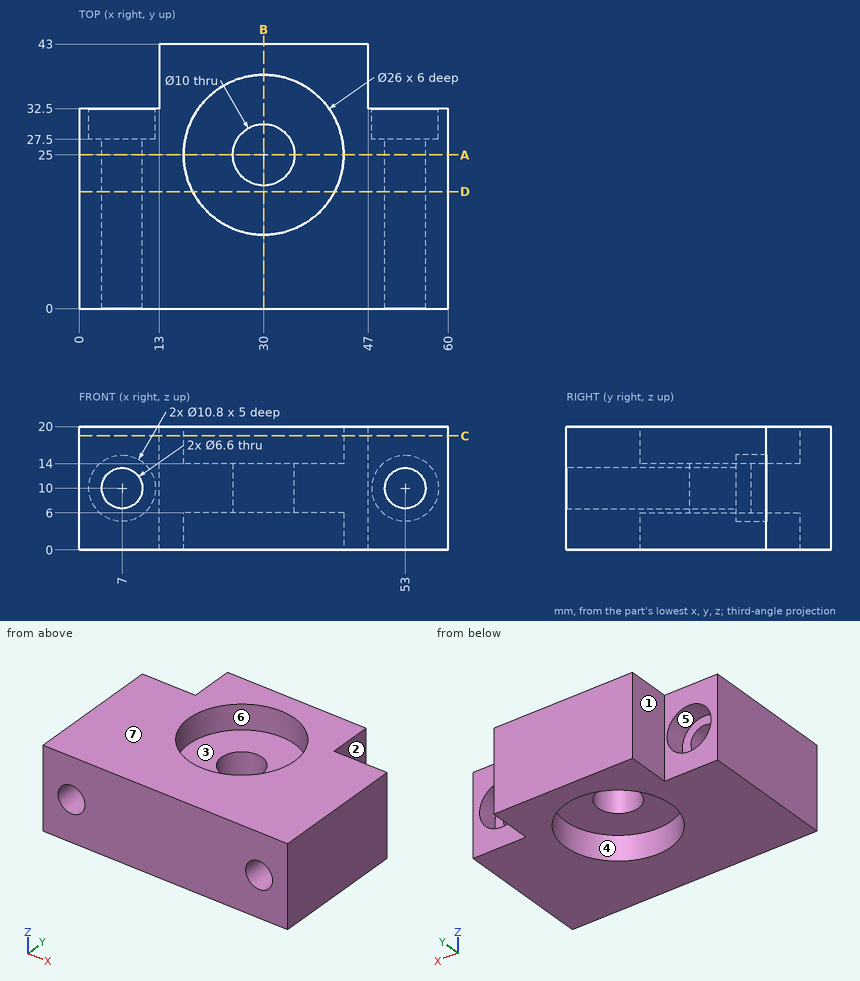
Design review of the part shown in the three views and the two pictorial views. Dimensions are in mm from the part's minimum x, y and z. A direction names the side the tool comes from. Round coordinates to 2 decimals unless told otherwise and drop trailing zeros. Order: outer loops, then holes, each group sorted by start corner. A loop starts at its lowest first (then second) coordinate and runs counter-clockwise, first axis right, second up. Notation, with made-up numbers: (-25.75, 82.25) -> (20.25, 82.25) arc R12 ccw to (20.25, 94.25) -> close; hole circle Ø5 at (47.5, -15.75). An arc over 180 degrees is marked (long way). Write item = value, one per line. Start each with the question number.
1) Insertion check: pin 1 (6 mm diameter, centred on x = 30, y = 25, fed in from +Z); pin 2 (3 mm diameter, centred on x = 26, y = 24, fed in from +Z); pin 3 (1 mm diameter, centred on x = 53, z = 6, fed in from +Y); pin 4 (3 mm diameter, centred on y = 39, z = 8, fed in from +X). Each pin has a flat end and moves straight along its axis. Give the tip position at first contact, or say it passes through.
2) To check wall thickness, follow line 1 (X direction, y = 25, z = 10.25); line 2 (Y direction, x = 30, z = 8.75); line 3 (Y direction, x = 55, z = 2). State the ranges of each line that lie inside material, in increasing order. Write a range as from..to.
3) Tool access review of the marked faces 1, 2, 3 and 4: name each direction out of +Z, -Z, +X, -X, +Y, -Y from which nothing blocks a thin tool from reaching the whole face with its end or side.
4) Take a section at D-D on y = 19. State the section outline as (x, z) points, plus the area to 3 significant figures.
5) Take a section at A-A on y = 25. State the section outline as (x, z) points, plus the area to 3 significant figures.
6) Take a section at B-B on x = 30. State the section outline as (y, z) points, plus the area to 3 significant figures.
7) Take a section at C-C on z = 18.5. State the section outline as (x, y) points.
8) The part is to be moulded in two halves that separate along Z. For the marked faces 5, 6 and 7, say which applies: +Z half, -Z half, draft (parallel to the pull), parting line (faces both ways), or undercut.
Verdict:
q1.pin_1 = through
q1.pin_2 = 14
q1.pin_3 = 27.5
q1.pin_4 = 47
q2.line_1 = 0..3.71, 10.29..25, 35..49.71, 56.29..60
q2.line_2 = 0..20, 30..43
q2.line_3 = 0..32.5
q3.face_1 = +Z, -Z, -X, +Y
q3.face_2 = +Z, -Z, +X, +Y
q3.face_3 = +Z
q3.face_4 = -Z
q4.outline = (0, 0) -> (18.47, 0) -> (18.47, 6) -> (41.53, 6) -> (41.53, 0) -> (60, 0) -> (60, 20) -> (41.53, 20) -> (41.53, 14) -> (18.47, 14) -> (18.47, 20) -> (0, 20) -> close; hole circle Ø6.6 at (7, 10); hole circle Ø6.6 at (53, 10)
q4.area = 855 mm2
q5.outline = (0, 0) -> (17, 0) -> (17, 6) -> (25, 6) -> (25, 14) -> (17, 14) -> (17, 20) -> (0, 20) -> close; (35, 6) -> (43, 6) -> (43, 0) -> (60, 0) -> (60, 20) -> (43, 20) -> (43, 14) -> (35, 14) -> close; hole circle Ø6.6 at (7, 10); hole circle Ø6.6 at (53, 10)
q5.area = 740 mm2
q6.outline = (0, 0) -> (12, 0) -> (12, 6) -> (20, 6) -> (20, 14) -> (12, 14) -> (12, 20) -> (0, 20) -> close; (30, 6) -> (38, 6) -> (38, 0) -> (43, 0) -> (43, 20) -> (38, 20) -> (38, 14) -> (30, 14) -> close
q6.area = 468 mm2
q7.outline = (0, 0) -> (60, 0) -> (60, 32.5) -> (47, 32.5) -> (47, 43) -> (13, 43) -> (13, 32.5) -> (0, 32.5) -> close; hole circle Ø26 at (30, 25)
q8.face_5 = undercut
q8.face_6 = draft
q8.face_7 = +Z half
